from build123d import *

# Parameters (mm, degrees)
F1_DEPTH    = 10
F2_T1_DEPTH = 25
F2_T3_DEPTH = 24.1421356237
F2_T5_DEPTH = 19.0165664987
F2_T7_DEPTH = 13.7370663506
F3_R        = 1
F4_T1_DEPTH = 10
F4_T3_DEPTH = 10
F4_T5_DEPTH = 22.9903810568


# Not quite as in the source:
# - a fillet or chamfer that OpenCascade refuses, or shapes differently, is made with other operations: its cross-section is extruded or revolved along the edge and cut away or added
# - a feature names something its author has since deleted; it is built from what else it names


with BuildPart() as f1:
    # F0 (on Front) → F1 (new body)
    with BuildSketch(Plane.XZ):
        Polygon((-50, 8.2), (-35, 8.2), (-35, 10.2), (-53, 10.2), (-53, -68.2), (-49, -68.2), (-49, -63.2), (-48.5, -63.2), (-48.5, -8.2), (-50, -8.2), align=None)
        Polygon((-49, -68.2), (-53, -68.2), (-44.5, -84.2), (-40.5, -84.2), align=None)
        Polygon((-12, -74.2), (-15, -74.2), (-15, -84.2), (-40.5, -84.2), (-44.5, -84.2), (-42.90625, -87.2), (-12, -87.2), align=None)
        Polygon((-40.5, -68.2), (-40.5, -63.2), (-48.5, -63.2), (-49, -63.2), (-49, -68.2), align=None)
    extrude(amount=F1_DEPTH)

    # F2: fillet of radius 3 on 6 edges, made by hand

    # F2_s2 → F2_t1 (cut)
    with BuildSketch(Plane.XZ.offset(-7.5)):
        with BuildLine():
            ThreePointArc((-50, 10.2), (-52.1213203436, 9.3213203436), (-53, 7.2))
            Line((-53, 7.2), (-53, 10.2))
            Line((-53, 10.2), (-50, 10.2))
        make_face()
        with BuildLine():
            ThreePointArc((-12, -77.2), (-12.8786796564, -75.0786796564), (-15, -74.2))
            Line((-15, -74.2), (-12, -74.2))
            Line((-12, -74.2), (-12, -77.2))
        make_face()
        with BuildLine():
            ThreePointArc((-15, -87.2), (-12.8786796564, -86.3213203436), (-12, -84.2))
            Line((-12, -84.2), (-12, -87.2))
            Line((-12, -87.2), (-15, -87.2))
        make_face()
    extrude(amount=F2_T1_DEPTH, mode=Mode.SUBTRACT)

    # F2_s4 → F2_t3 (cut)
    with BuildSketch(Plane.XZ.offset(-7.0710678119)):
        with BuildLine():
            ThreePointArc((-35, 8.2), (-36.0963763172, 9.6494897428), (-37.8284271247, 10.2))
            Line((-37.8284271247, 10.2), (-35, 10.2))
            Line((-35, 10.2), (-35, 8.2))
        make_face()
    extrude(amount=F2_T3_DEPTH, mode=Mode.SUBTRACT)

    # F2_s6 → F2_t5 (cut)
    with BuildSketch(Plane.XZ.offset(-4.5082832494)):
        with BuildLine():
            ThreePointArc((-43.7522838586, -85.6074656779), (-42.648511507, -86.7712251004), (-41.1029367003, -87.2))
            Line((-41.1029367003, -87.2), (-42.90625, -87.2))
            Line((-42.90625, -87.2), (-43.7522838586, -85.6074656779))
        make_face()
    extrude(amount=F2_T5_DEPTH, mode=Mode.SUBTRACT)

    # F2_s8 → F2_t7 (cut)
    with BuildSketch(Plane.XZ.offset(-1.8685331753)):
        with BuildLine():
            ThreePointArc((-53, -67.4525867299), (-52.9110171311, -68.1778310077), (-52.6493471584, -68.8600524078))
            Line((-52.6493471584, -68.8600524078), (-53, -68.2))
            Line((-53, -68.2), (-53, -67.4525867299))
        make_face()
    extrude(amount=F2_T7_DEPTH, mode=Mode.SUBTRACT)

    # F3
    f3_edges = [f1.edges().sort_by_distance(p)[0] for p in [
        (-40.5, -5, -84.2),
        (-15, -5, -84.2),
        (-50, -5, 8.2),
    ]]
    fillet(f3_edges, radius=F3_R)

    # F4: fillet of radius 3 on 3 edges, made by hand

    # F4_s2 → F4_t1 (join)
    with BuildSketch(Plane.XZ):
        with BuildLine():
            ThreePointArc((-46.6585338586, -72.6074656779), (-46.5804118006, -69.6544251933), (-44.0091867003, -68.2))
            Line((-44.0091867003, -68.2), (-49, -68.2))
            Line((-49, -68.2), (-46.6585338586, -72.6074656779))
        make_face()
    extrude(amount=F4_T1_DEPTH)

    # F4_s4 → F4_t3 (join)
    with BuildSketch(Plane.XZ):
        with BuildLine():
            ThreePointArc((-45.5, -63.2), (-47.6213203436, -62.3213203436), (-48.5, -60.2))
            Line((-48.5, -60.2), (-48.5, -63.2))
            Line((-48.5, -63.2), (-45.5, -63.2))
        make_face()
    extrude(amount=F4_T3_DEPTH)

    # F4_s6 → F4_t5 (cut)
    with BuildSketch(Plane.XZ.offset(-6.4951905284)):
        with BuildLine():
            ThreePointArc((-50, -8.2), (-48.9019237886, -9.2980762114), (-48.5, -10.7980762114))
            Line((-48.5, -10.7980762114), (-48.5, -8.2))
            Line((-48.5, -8.2), (-50, -8.2))
        make_face()
    extrude(amount=F4_T5_DEPTH, mode=Mode.SUBTRACT)


solid = f1.part
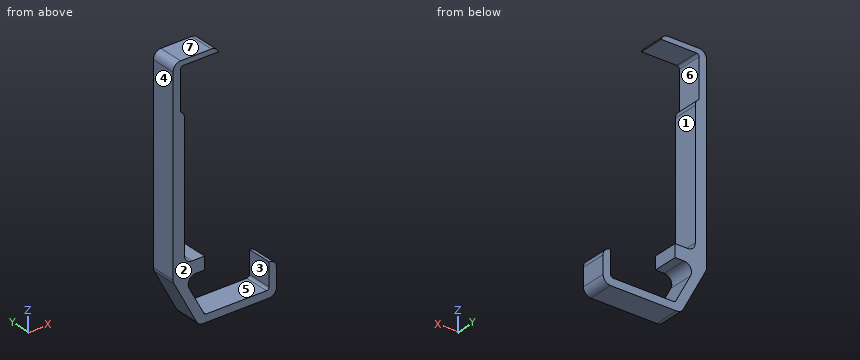
Geometry check sheet. Reference: the model listing, model coordinates, mm. Face numbers are marked on the shaded views. A direction names the side the tool comes from. Give positions to 0.01 mm unless a question says otherwise; leave off trailing zeros. Loops run counter-clockwise (first coordinate to the right, second up) from the corner with the lowest first, then second, coordinate; pieces in that order, holes last. Notation, with made-up numbers: M 15.25,-30.5 L 67.25,-30.5 A23 cw 67.25,-18.5 Z; hole C -29,24.25 d1. An arc over 180 degrees is marked long. Write each question's results on one line, items separated by ' | '.
1) Section check C-C, the plane z = -19. Record the boundary of the cut face in (x, y).
Answers follow:
outline: M -53,-10 L -48.5,-10 L -48.5,0 L -53,0 Z
2) Gauge pin test, flat ends, axial feed: pin 1 (1.1 mm diameter, centred on x = -42.5, y = -7, fed in from -Z); pin 2 (2 mm diameter, centred on y = -3.5, z = -41, fed in from +X); pin 3 (5 mm diameter, centred on y = -2.5, z = 2, fed in from +X). Record the tip position at first contact, or that the pin passes through.
Answers follow:
pin 1: z = -87.08 | pin 2: x = -48.5 | pin 3: x = -50
3) Section check B-B, the plane x = -30. Record the boundary of the cut face in (y, z).
Answers follow:
outline: M -10,-87.2 L 0,-87.2 L 0,-84.2 L -10,-84.2 Z
4) Release check for a two-part mould opening along Z. For the marked faces 4, 5, 6 and 7 record: +Z half, -Z half, draft (parallel to the pull), parting line (faces both ways), or undercut.
Answers follow:
face 4: draft | face 5: undercut | face 6: undercut | face 7: +Z half
5) Tool access check on the marked faces 1, 2 and 3. Record the directions out of +Z, -Z, +X, -X, +Y, -Y that give a thin tool (end or side, any length) a straight path to the whole face; none if there is none.
Answers follow:
face 1: +X, +Y, -Y | face 2: +Z, -Z, +X, -X, -Y | face 3: +Z, +Y, -Y
6) Section check A-A, the plane y = -7.5. Record the boundary of the cut face in (x, z), plus the area to 3 significant figures.
Answers follow:
outline: M -53,-67.45 A3 ccw -52.65,-68.86 L -43.75,-85.61 A3 ccw -41.1,-87.2 L -15,-87.2 A3 ccw -12,-84.2 L -12,-77.2 A3 ccw -15,-74.2 L -15,-83.2 A1 cw -16,-84.2 L -39.9,-84.2 A1 cw -40.78,-83.67 L -46.66,-72.61 A3 cw -44.01,-68.2 L -40.5,-68.2 L -40.5,-63.2 L -45.5,-63.2 A3 cw -48.5,-60.2 L -48.5,-10.8 A3 ccw -50,-8.2 L -50,7.2 A1 cw -49,8.2 L -35,8.2 A3 ccw -37.83,10.2 L -50,10.2 A3 ccw -53,7.2 Z | area: 583 mm2
7) Thickness scan on line 1 (Z direction, x = -41, y = -6); line 2 (X direction, y = -9, z = 0); line 3 (Z direction, x = -32, y = -5.75). Record the ranges inside material, lowest first.
Answers follow:
line 1: -87.2 to -83.26, -68.2 to -63.2, 8.2 to 10.2 | line 2: -53 to -50 | line 3: -87.2 to -84.2
